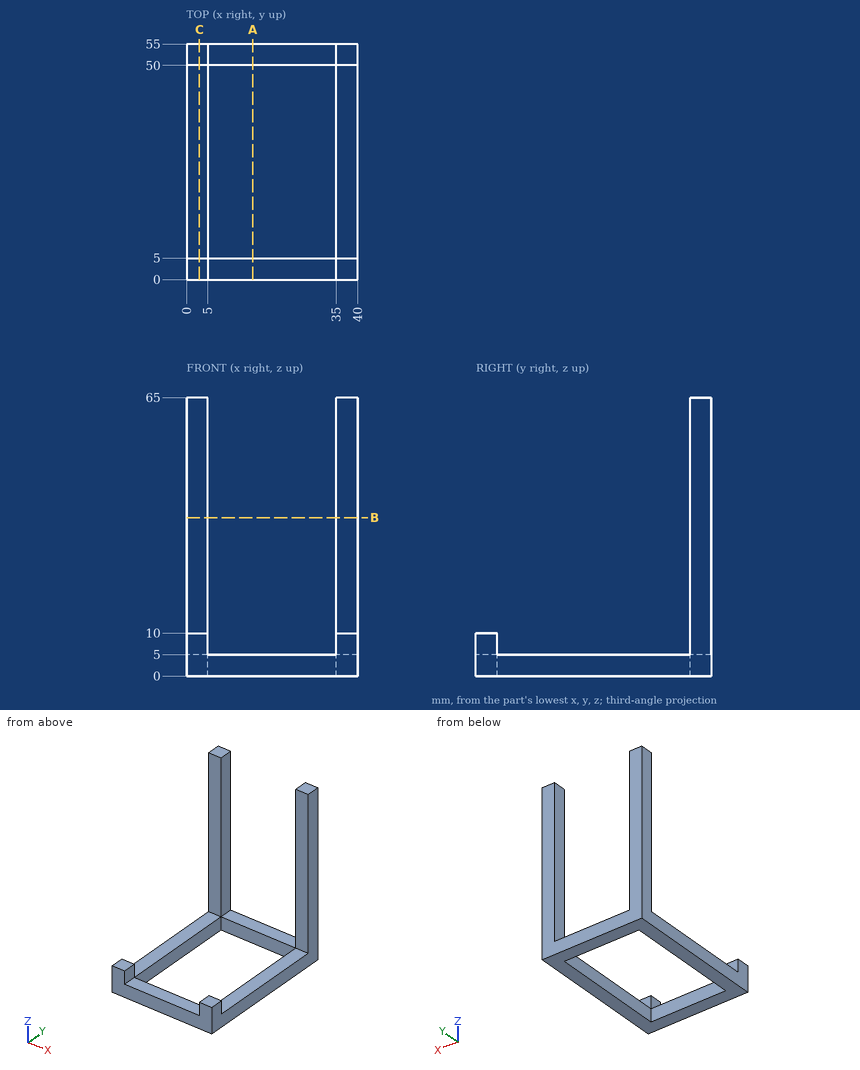
Geometry check sheet. Reference: drawing and pictorial views, mm from the part's lowest x, y, z. Round coordinates to 2 decimals unless told otherwise and drop trailing zeros. Order: outer loops, then holes, each group sorted by start corner. A loop starts at its lowest first (then second) coordinate and runs counter-clockwise, first axis right, second up. Notation, with made-up numbers: M -17,-24.75 L 40,-24.75 A8 cw 40,-20.75 Z; hole C -14.75,-8 d3. An arc over 180 degrees is marked long. Write item = value, one per line.
Q1. Section check B-B (z = 37). Enter the section's corners in (x, y), plus the area to 3 significant figures.
Answer block:
outline = M 0,50 L 5,50 L 5,55 L 0,55 Z; M 35,50 L 40,50 L 40,55 L 35,55 Z
area = 50.0 mm^2
Q2. Depth check by flat-ended pin: pin 1 Ø4 at (x, z) = (2, 28.5) entering from -Y; pin 2 Ø1 at (x, z) = (22.5, 7) entering from +Y; pin 3 Ø5.5 at (x, y) = (2.5, 37) entering from +Z; pin 4 Ø2.5 at (x, y) = (37.5, 3) entering from +Z. Enter the tip coordinate at first touch or a pass-through.
Answer block:
pin_1 = 50
pin_2 = through
pin_3 = 5
pin_4 = 10
Q3. Scan lines: line 1 (X direction, y = 53.5, z = 6); line 2 (Y direction, x = 4.5, z = 7); line 3 (Z direction, x = 21.5, y = 4). Record each from-to range of solid material in increasing order.
Answer block:
line_1 = 0 to 5, 35 to 40
line_2 = 0 to 5, 50 to 55
line_3 = 0 to 5
Q4. Section check C-C (x = 3). Enter the section's corners in (y, z), plus the area to 3 significant figures.
Answer block:
outline = M 0,0 L 55,0 L 55,65 L 50,65 L 50,5 L 5,5 L 5,10 L 0,10 Z
area = 600 mm^2
Q5. Section check A-A (x = 15.5). Enter the section's corners in (y, z).
Answer block:
outline = M 0,0 L 5,0 L 5,5 L 0,5 Z; M 50,0 L 55,0 L 55,5 L 50,5 Z
